Check sheet for the modelled part. Datum: model origin and axes. Units: mm. Face numbers are marked on the shaded views. A direction names the side the tool comes from. Round coordinates to 2 decimals unless told otherwise and drop trailing zeros. Write each loop counter-clockwise with the first axis right and the second up, starting at its lowest first coordinate (ties: lowest second). Pieces come first, ordered by that corner, then holes.
Item 1: Go/stop test with flat-tipped pins: pin 1 Ø1.9 at (x, y) = (-5, -3) entering from -Z; pin 2 Ø0.9 at (y, z) = (-6, 2.5) entering from +X; pin 3 Ø2 at (x, y) = (-2, 6.5) entering from -Z; pin 4 Ø1.8 at (x, z) = (-4, 2.5) entering from -Y. Record where each tip stops, or that it passes through.
Item 2: Cross-section at A-A on y = -6.25. Enter the section's corners in (x, z), plus the area to 3 significant figures.
Item 3: Cross-section at D-D on x = 3.5. Enter the section's corners in (y, z).
Item 4: Material ranges on line 1 (Y direction, x = 7.25, z = 0.8); line 2 (Y direction, x = -5.5, z = 0.65), recorded low to high.
Item 5: Cross-section at B-B on z = 5.45. Enter the section's corners in (x, y), plus the area to 3 significant figures.
Item 6: Cross-section at C-C on x = -5. Enter the section's corners in (y, z).
Item 7: Release check for a two-part mould opening along Y. For the marked faces 1, 2, 3 and 4 record: +Y half, -Y half, draft (parallel to the pull), parting line (faces both ways), or undercut.
Item 8: Tool access check on the marked faces 5, 6, 7, 8 and 9. Record the directions out of +Z, -Z, +X, -X, +Y, -Y that give a thin tool (end or side, any length) a straight path to the whole face; none if there is none.
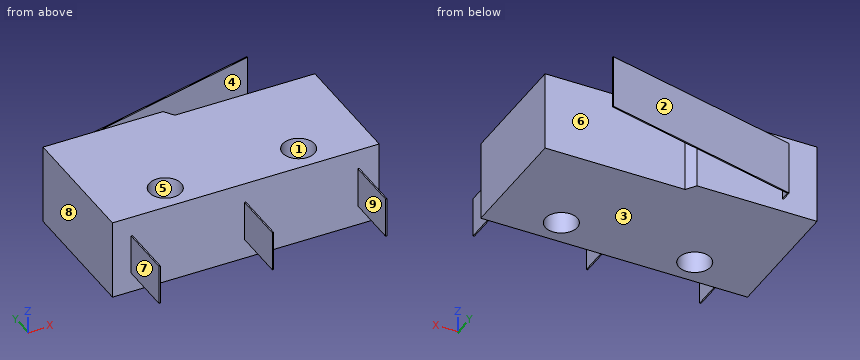
from build123d import *

# Parameters (mm, degrees)
SKETCH1_R           = 1.2
BOSS_EXTRUDE1_DEPTH = 6
EXTRUDE_THIN1_START = -1
EXTRUDE_THIN1_DEPTH = 4
SKETCH3_W           = 0.1
SKETCH3_H           = 3
EXTRUDE_THIN2_DEPTH = 4


with BuildPart() as part:
    # Sketch1 → Boss-Extrude1 (new body)
    with BuildSketch(Plane.XY):
        Polygon((-0.5, 4.258314247), (-1, 5), (-10, 5), (-10, -5), (10, -5), (10, 4.258314247), align=None)
        with Locations((-5, -3)):
            Circle(SKETCH1_R, mode=Mode.SUBTRACT)
        with Locations((5, -3)):
            Circle(SKETCH1_R, mode=Mode.SUBTRACT)
    extrude(amount=BOSS_EXTRUDE1_DEPTH)

    # Sketch2 → Extrude-Thin1 (add)
    with BuildSketch(Plane.XY.offset(6).offset(EXTRUDE_THIN1_START)):
        Polygon((-7.5, 5), (-7.5, 5.8), (7.571733766, 9.41840314), (7.595078303, 9.321166148), (-7.4, 5.721166357), (-7.4, 5), align=None)
    extrude(amount=-EXTRUDE_THIN1_DEPTH)

    # Sketch3 → Extrude-Thin2 (add)
    with BuildSketch(Plane.XZ.offset(5)):
        with Locations((-8.55, 3)):
            Rectangle(SKETCH3_W, SKETCH3_H)
        with Locations((8.45, 3)):
            Rectangle(SKETCH3_W, SKETCH3_H)
        with Locations((-0.05, 3)):
            Rectangle(SKETCH3_W, SKETCH3_H)
    extrude(amount=EXTRUDE_THIN2_DEPTH)


solid = part.part
Response values:
1. pin 1: passes through
1. pin 2: stops at x = 8.5
1. pin 3: stops at z = 1
1. pin 4: stops at y = -5
2. outline: (-8.6, 1.5) - (-8.5, 1.5) - (-8.5, 4.5) - (-8.6, 4.5) - close; (-0.1, 1.5) - (0, 1.5) - (0, 4.5) - (-0.1, 4.5) - close; (8.4, 1.5) - (8.5, 1.5) - (8.5, 4.5) - (8.4, 4.5) - close
2. area: 0.900 mm2
3. outline: (-5, 0) - (4.26, 0) - (4.26, 6) - (-5, 6) - close; (8.34, 1) - (8.44, 1) - (8.44, 5) - (8.34, 5) - close
4. line 1: y = -5 to 4.26
4. line 2: y = -5 to -4.09, -1.91 to 5
5. outline: (-10, -5) - (10, -5) - (10, 4.26) - (-0.5, 4.26) - (-1, 5) - (-10, 5) - close; hole circle Ø2.4 at (-5, -3); hole circle Ø2.4 at (5, -3)
5. area: 183 mm2
6. outline: (-5, 0) - (-4.2, 0) - (-4.2, 6) - (-5, 6) - close; (-1.8, 0) - (5, 0) - (5, 6) - (-1.8, 6) - close; (6.3, 1) - (6.4, 1) - (6.4, 5) - (6.3, 5) - close
7. face 1: undercut
7. face 2: +Y half
7. face 3: draft
7. face 4: undercut
8. face 5: +Z, -Z
8. face 6: +Z, -Z, +X
8. face 7: +Z, -Z, -X, -Y
8. face 8: +Z, -Z, -X, +Y, -Y
8. face 9: +Z, -Z, -Y
